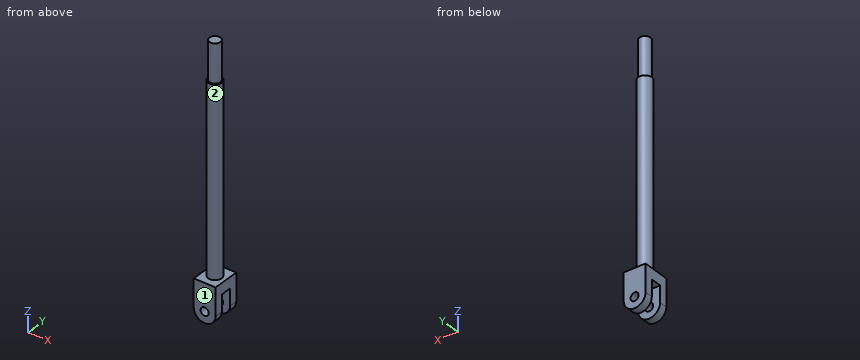
from build123d import *

# Parameters (mm, degrees)
F0_R     = 3.96875
F1_DEPTH = 107.95
F2_R     = 3.175
F3_DEPTH = 22.225
F4_R     = 2.361553
F5_DEPTH = 7.9375
F7_DEPTH = 3.175


with BuildPart() as f1:
    # F0 (on Top) → F1 (new body)
    with BuildSketch(Plane.XY):
        Circle(F0_R)
    extrude(amount=F1_DEPTH)

    # F2 (on face) → F3 (join)
    with BuildSketch(Plane.XY.offset(107.95)):
        Circle(F2_R)
    extrude(amount=F3_DEPTH)

    # F4 (on Front) → F5 (join, symmetric)
    with BuildSketch(Plane.XZ):
        with BuildLine():
            Line((3.96875, 0), (-3.96875, 0))
            Line((-3.96875, 0), (-6.35, 0))
            Line((-6.35, 0), (-6.35, -15.875))
            ThreePointArc((-6.35, -15.875), (0, -22.225), (6.35, -15.875))
            Line((6.35, -15.875), (6.35, 0))
            Line((6.35, 0), (3.96875, 0))
        make_face()
        with Locations((0, -15.875)):
            Circle(F4_R, mode=Mode.SUBTRACT)
    extrude(amount=F5_DEPTH, both=True)

    # F6 (on Front) → F7 (cut, symmetric)
    with BuildSketch(Plane.XZ):
        with BuildLine():
            Line((6.35, -15.875), (6.35, -6.35))
            Line((6.35, -6.35), (-6.35, -6.35))
            Line((-6.35, -6.35), (-6.35, -15.875))
            ThreePointArc((-6.35, -15.875), (0, -22.225), (6.35, -15.875))
        make_face()
    extrude(amount=F7_DEPTH, both=True, mode=Mode.SUBTRACT)


solid = f1.part
The listing builds one solid part. Answer for the finished solid, in the listing's coordinates (mm). Face numbers are marked on the shaded views. A direction names the side the tool comes from. Coordinates: 2 decimals unless noted, no trailing zeros. Loops run counter-clockwise (first coordinate to the right, second up) from the corner with the lowest first, then second, coordinate; pieces in that order, holes last. Notation, with made-up numbers: (-37, -26) -> (8, -26) arc R25 cw to (8, 7) -> close; hole circle Ø4 at (27.5, 5). An arc over 180 degrees is marked (long way). Answer in a Markdown table with one row per item. Add a question column.
1. For the marked faces 1 and 2, determine the directions among +Z, -Z, +X, -X, +Y, -Y from which every point of the face is accessible in a straight line to the end or side of a thin tool.
2. Consider line 1 (Y direction, x = -4, z = -12.5) (1 decimal); line 2 (Z direction, x = 0, y = -5.5) (3 decimals); line 3 (Z direction, x = -2, y = -2.5). Determine where each line is inside the solid, lowest interval first. Write a range as [from, to].
3. The part is cut by section B-B, the plane y = -6.25. Write down the section's boundary in (x, z) (3 decimals).
4. The part is cut by section A-A, the plane x = 0. Count the separate pieces of the cut face and the enclosed holes in it, then the cut area to 3 significant figures.
5. Flat-ended cylindrical pins translate along their axes: P1, Ø1.5, axis at y = 2.5, z = 76.5, coming from the +X side; P2, Ø1.9, axis at x = 0.5, y = 1.5, coming from the -Z side; P3, Ø4, axis at x = -3, z = 64.5, coming from the +Y side. Find the tip coordinate at first contact, or state that the pin passes through.
6. The part is cut by section C-C, the plane y = 0. Write down the section's boundary in (x, z) (3 decimals).
7. The part is cut by section D-D, the plane z = 114.5. Write down the section's boundary in (x, y) (3 decimals), then the cut area to 3 significant figures.
Answer below:
| question | item | result |
|---|---|---|
| 1 | face 1 | +Z, -Z, +X, -X, -Y |
| 1 | face 2 | +Z |
| 2 | line 1 | [-7.9, -3.2], [3.2, 7.9] |
| 2 | line 2 | [-22.225, -18.237], [-13.513, 0] |
| 2 | line 3 | [-6.35, 107.95] |
| 3 | outline | (-6.35, -15.875) arc R6.35 ccw to (6.35, -15.875) -> (6.35, 0) -> (-6.35, 0) -> close; hole circle Ø4.723 at (0, -15.875) |
| 4 | separate pieces | 3 |
| 4 | enclosed holes | 0 |
| 4 | area | 1,210 mm2 |
| 5 | P1 | x = 3.56 |
| 5 | P2 | z = -6.35 |
| 5 | P3 | y = 3.84 |
| 6 | outline | (-6.35, -6.35) -> (6.35, -6.35) -> (6.35, 0) -> (3.969, 0) -> (3.969, 107.95) -> (3.175, 107.95) -> (3.175, 130.175) -> (-3.175, 130.175) -> (-3.175, 107.95) -> (-3.969, 107.95) -> (-3.969, 0) -> (-6.35, 0) -> close |
| 7 | outline | circle Ø6.35 at (0, 0) |
| 7 | area | 31.7 mm2 |
